Work out the finished part from the listing and answer in its coordinate system (mm). A direction names the side the tool comes from. Round coordinates to 2 decimals unless told otherwise and drop trailing zeros. Order: outer loops, then holes, each group sorted by start corner. A loop starts at its lowest first (then second) coordinate and runs counter-clockwise, first axis right, second up. Notation, with made-up numbers: M 41,19.5 L 96,19.5 A17 cw 96,24.5 Z; hole C 15,71 d3. An arc over 180 degrees is marked long. Return JSON: item names as keys, results as strings.
from build123d import *

# Parameters (mm, degrees)
PROFILESKETCH3_W                           = 15
PROFILESKETCH3_H                           = 21.85
PROFILEBOSS_EXTRUDE1_DEPTH                 = 9
MICROSWITCHCUTSKETCH4_W                    = 12.05
MICROSWITCHCUTSKETCH4_H                    = 13.05
MICROSWITCHCUT_EXTRUDE1_DEPTH              = 4.8
SKETCH5_R                                  = 1.55
MICROSWITCHMOUNTINGHOLESCUT_EXTRUDE2_DEPTH = 3.1
SMALLCHANNELCABLESKETCH6_W                 = 2.95
SMALLCHANNELCABLESKETCH6_H                 = 1.75
SMALLCHANNELCABLECUT_EXTRUDE3_DEPTH        = 4.75
LARGECHANNELCABLESKETCH7_W                 = 2.95
LARGECHANNELCABLESKETCH7_H                 = 3.75
LARGECHANNELCABLECUT_EXTRUDE4_DEPTH        = 1.75
CHAMFER1_SIZE                              = 1
SKETCH6_R                                  = 2.5
MICROSWITCHMOUNTINGHOLECUT_EXTRUDE1_DEPTH  = 28.9896856


with BuildPart() as part:
    # ProfileSketch3 → ProfileBoss-Extrude1 (new body)
    with BuildSketch(Plane.XY):
        with Locations((7.5, 10.925)):
            Rectangle(PROFILESKETCH3_W, PROFILESKETCH3_H)
    extrude(amount=PROFILEBOSS_EXTRUDE1_DEPTH)

    # MicroSwitchCutSketch4 → MicroSwitchCut-Extrude1 (cut)
    with BuildSketch(Plane.XY.offset(9)):
        with Locations((6.025, 6.525)):
            Rectangle(MICROSWITCHCUTSKETCH4_W, MICROSWITCHCUTSKETCH4_H)
    extrude(amount=-MICROSWITCHCUT_EXTRUDE1_DEPTH, mode=Mode.SUBTRACT)

    # Sketch5 → MicroSwitchMountingHolesCut-Extrude2 (cut)
    with BuildSketch(Plane.XY.offset(4.2)):
        with Locations((5.05, 9.7)):
            Circle(SKETCH5_R)
        with Locations((5.05, 3.35)):
            Circle(SKETCH5_R)
    extrude(amount=-MICROSWITCHMOUNTINGHOLESCUT_EXTRUDE2_DEPTH, mode=Mode.SUBTRACT)

    # SmallChannelCableSketch6 → SmallChannelCableCut-Extrude3 (cut)
    with BuildSketch(Plane.XY.offset(9)):
        with Locations((13.525, 6.525)):
            Rectangle(SMALLCHANNELCABLESKETCH6_W, SMALLCHANNELCABLESKETCH6_H)
    extrude(amount=-SMALLCHANNELCABLECUT_EXTRUDE3_DEPTH, mode=Mode.SUBTRACT)

    # LargeChannelCableSketch7 → LargeChannelCableCut-Extrude4 (cut)
    with BuildSketch(Plane.XY.offset(4.25)):
        with Locations((13.525, 6.525)):
            Rectangle(LARGECHANNELCABLESKETCH7_W, LARGECHANNELCABLESKETCH7_H)
    extrude(amount=-LARGECHANNELCABLECUT_EXTRUDE4_DEPTH, mode=Mode.SUBTRACT)

    # Chamfer1
    chamfer1_edges = [part.edges().sort_by_distance(p)[0] for p in [
        (12.05, 6.525, 4.2),
    ]]
    chamfer(chamfer1_edges, length=CHAMFER1_SIZE)

    # Sketch6 → MicroSwitchMountingHoleCut-Extrude1 (cut, through all)
    with BuildSketch(Plane.XY.offset(9)):
        with Locations((7.5, 16.35)):
            Circle(SKETCH6_R)
    extrude(amount=-MICROSWITCHMOUNTINGHOLECUT_EXTRUDE1_DEPTH, mode=Mode.SUBTRACT)


solid = part.part
Item 1: Find section D-D (y = 3.35). Determine the outline of the cut face in (x, z).
Output:
{"outline": "M 0,0 L 15,0 L 15,9 L 12.05,9 L 12.05,4.2 L 6.6,4.2 L 6.6,1.1 L 3.5,1.1 L 3.5,4.2 L 0,4.2 Z"}
Item 2: The mould has two halves that part along Y. Classify faces 4 (the cylindrical face through (6.528, 3.816, 2.672)), 5 (the flat face through (11, 16, 9)), 6 (the flat face through (6, 13.05, 7)): pulls with the +Y half, pulls with the -Y half, needs draft (parallel to the pull), parting line crosses it, or undercut.
Output:
{"face 4": "undercut", "face 5": "needs draft", "face 6": "pulls with the -Y half"}
Item 3: Consider line 1 along Y through (x, z) = (7.5, 5.5); line 2 along Z through (x, y) = (9, 8.75); line 3 along X through (y, z) = (3, 2). Determine where each line is inside the solid, lowest interval first. Write a range as [from, to].
Output:
{"line 1": "y = [13.05, 13.85], [18.85, 21.85]", "line 2": "z = [0, 4.2]", "line 3": "x = [0, 3.54], [6.56, 15]"}
Item 4: Each of these flat-tipped pins is pushed along its axis until it touches: pin 1 (1.5 mm diameter, centred on x = 5, y = 10, fed in from +Z); pin 2 (2.5 mm diameter, centred on x = 5.5, z = 7.5, fed in from -Y); pin 3 (3.5 mm diameter, centred on x = 4.5, y = 4, fed in from +Z). Where does it stop, or does it pass through?
Output:
{"pin 1": "stops at z = 1.1", "pin 2": "stops at y = 13.05", "pin 3": "stops at z = 4.2"}
Item 5: Which of the six approach directions +Z, -Z, +X, -X, +Y, -Y give full straight-line access (tool end or side, diameter ignored) to faces 1 (the flat face through (14, 7.4, 7)), 2 (the flat face through (13, 4.65, 3)), 3 (the cylindrical face through (5.88, 11.01, 2.67))?
Output:
{"face 1": "+Z, +X, -X", "face 2": "+X", "face 3": "+Z"}
Item 6: Find section B-B (x = 7.5). Determine the outline of the cut face in (y, z).
Output:
{"outline": "M 0,0 L 13.85,0 L 13.85,9 L 13.05,9 L 13.05,4.2 L 0,4.2 Z; M 18.85,0 L 21.85,0 L 21.85,9 L 18.85,9 Z"}
Item 7: Find section A-A (z = 2). Determine the outline of the cut face in (x, y), plus the area to 3 significant figures.
Output:
{"outline": "M 0,0 L 15,0 L 15,21.85 L 0,21.85 Z; hole C 5.05,3.35 d3.1; hole C 5.05,9.7 d3.1; hole C 7.5,16.35 d5", "area": "293 mm^2"}
Item 8: Find section C-C (y = 16.35). Determine the outline of the cut face in (x, z), plus the area to 3 significant figures.
Output:
{"outline": "M 0,0 L 5,0 L 5,9 L 0,9 Z; M 10,0 L 15,0 L 15,9 L 10,9 Z", "area": "90.0 mm^2"}
